Source: CAD feature listing. Evaluate the final solid. Frame: model axes, mm. A direction names the side the tool comes from. Give positions to 0.01 mm unless a question says otherwise; leave off trailing zeros. Write each loop counter-clockwise with the first axis right and the second up, starting at its lowest first coordinate (ties: lowest second). Pieces come first, ordered by that corner, then holes. Notation, with made-up numbers: (-32, 64.5) -> (-14, 64.5) arc R20 ccw to (-14, 88.5) -> close; hole circle Ø1 at (32.25, -30). An arc over 180 degrees is marked (long way). Write item = value, one per line.
from build123d import *

# Parameters (mm, degrees)
SKETCH_1_R      = 6.05
EXTRUDE_1_DEPTH = 5
SKETCH_7_R      = 7
EXTRUDE_6_DEPTH = 1
SKETCH_2_R      = 6.05
EXTRUDE_2_DEPTH = 4
EXTRUDE_3_DEPTH = 15
FILLET_1_R      = 2
SKETCH_5_R      = 5.5
EXTRUDE_4_DEPTH = 1
SKETCH_6_R      = 5.05
EXTRUDE_5_DEPTH = 3
FILLET_2_R      = 1


with BuildPart() as part:
    # 草图1 → 凸台-拉伸1 (new body)
    with BuildSketch(Plane.XY):
        Circle(SKETCH_1_R)
    extrude(amount=EXTRUDE_1_DEPTH)

    # 草图7 → 凸台-拉伸6 (add)
    with BuildSketch(Plane.XY.offset(5)):
        Circle(SKETCH_7_R)
    extrude(amount=-EXTRUDE_6_DEPTH)

    # 草图2 → 凸台-拉伸2 (add)
    with BuildSketch(Plane.XY.offset(5)):
        with Locations((0, 0.75)):
            Circle(SKETCH_2_R)
    extrude(amount=EXTRUDE_2_DEPTH)

    # 草图4 → 凸台-拉伸3 (add)
    with BuildSketch(Plane(origin=(0, 0, 0), x_dir=(-1, 0, 0), z_dir=(0, 0, -1))):
        with BuildLine():
            ThreePointArc((4, 0), (-1.645751311, 3.645751311), (-2.645751311, -3))
            Line((-2.645751311, -3), (2.645751311, -3))
            ThreePointArc((2.645751311, -3), (3.645751311, -1.645751311), (4, 0))
        make_face()
    extrude(amount=EXTRUDE_3_DEPTH)

    # 圆角1
    fillet_1_edges = [part.edges().sort_by_distance(p)[0] for p in [
        (0, -3, 0),
        (0, 4, 0),
    ]]
    fillet(fillet_1_edges, radius=FILLET_1_R)

    # 草图5 → 凸台-拉伸4 (add)
    with BuildSketch(Plane.XY.offset(9)):
        Circle(SKETCH_5_R)
    extrude(amount=EXTRUDE_4_DEPTH)

    # 草图6 → 凸台-拉伸5 (add)
    with BuildSketch(Plane.XY.offset(10)):
        Circle(SKETCH_6_R)
    extrude(amount=EXTRUDE_5_DEPTH)

    # 圆角2
    fillet_2_edges = [part.edges().sort_by_distance(p)[0] for p in [
        (-5.05, 0, 13),
    ]]
    fillet(fillet_2_edges, radius=FILLET_2_R)


solid = part.part
(1) Section query B-B (z = 10.75). Return loops of the section in (x, y), plus the area to 3 significant figures.
Values follow:
outline = circle Ø10.1 at (0, 0)
area = 80.1 mm2
(2) Material intervals for line 1 (X direction, y = -0.25, z = 3.5); line 2 (Z direction, x = -5.75, y = 1); line 3 (Z direction, x = 4, y = 4.75), sorted ascending.
Values follow:
line_1 = -6.04 to 6.04
line_2 = -0.01 to 9
line_3 = 4 to 9
(3) Section query C-C (z = -0.5). Return loops of the section in (x, y).
Values follow:
outline = (-2.89, -3.68) -> (2.89, -3.68) arc R4.68 ccw (long way) to start
(4) First-contact query: pin 1 (2 mm diameter, centred on y = -4.5, z = 6.5, fed in from +X); pin 2 (2.5 mm diameter, centred on x = -0.5, z = -8, fed in from -Y); pin 3 (0.8 mm diameter, centred on x = -1.5, y = -5, fed in from -Z). Flat tips, straight axial feed; report the tip coordinate or a pass-through.
Values follow:
pin_1 = 4.31
pin_2 = -3
pin_3 = -0.04
(5) Access query for faces 1 (the face through (0, -3, -8)), 2 (the face through (-1.19, -5.37, 9.49)), 3 (the face through (-0.5, -5.3, 0)). Directions: +Z, -Z, +X, -X, +Y, -Y. A direction counts if a zero-diameter tool reaches every point of the face in a straight line with its end or side. Return the directions, or none.
Values follow:
face_1 = -Z, +X, -X, -Y
face_2 = +Z
face_3 = -Z
(6) Section query A-A (z = -7.75). Return loops of the section in (x, y).
Values follow:
outline = (-2.65, -3) -> (2.65, -3) arc R4 ccw (long way) to start
(7) Pull-direction query (Z, two-part tool) for faces 4 (the face through (2.79, -4.62, 6.97)), 5 (the face through (4.817, 1.517, 10.986)), 6 (the face through (-2, 6, 4)), 7 (the face through (0, 6, 9)); classes: pulls with the +Z half, pulls with the -Z half, needs draft (parallel to the pull), parting line crosses it, or undercut.
Values follow:
face_4 = undercut
face_5 = needs draft
face_6 = pulls with the -Z half
face_7 = pulls with the +Z half
